Here's how the part is built. I have some questions about the finished solid (model axes, mm). Coordinates: 2 decimals unless noted, no trailing zeros. Write each loop counter-clockwise with the first axis right and the second up, starting at its lowest first coordinate (ties: lowest second). Pieces come first, ordered by that corner, then holes.
Item 1: I want a section at D-D (x = 50). Please give me the cut outline in (y, z), and give its area (3 significant figures).
Item 2: I'm going to push flat-ended pins straight in: P1, Ø3, axis at x = -8.49, y = -8.49, coming from the +Z side; P2, Ø1.5, axis at y = -23, z = 1.5, coming from the +X side; P3, Ø1.5, axis at x = -51, z = 3, coming from the +Y side; P4, Ø2, axis at x = -37.5, z = 3, coming from the -Y side. Where does each tip first touch, or does it pass through?
Item 3: I want a section at A-A (y = 0). Please give me the cut outline in (x, z), and give its area (4 significant figures).
Item 4: I want a section at C-C (y = -50). Please give me the cut outline in (x, z), and give its area (3 significant figures).
Item 5: Please list where these lines run through material, in increasing order: line 1 (Y direction, x = -39.5, z = 4.2); line 2 (Y direction, x = -14, z = 1.35); line 3 (Y direction, x = 1, z = 0.65).
Item 6: I want a section at B-B (x = 0). Please give me the cut outline in (y, z), and give its area (4 significant figures).
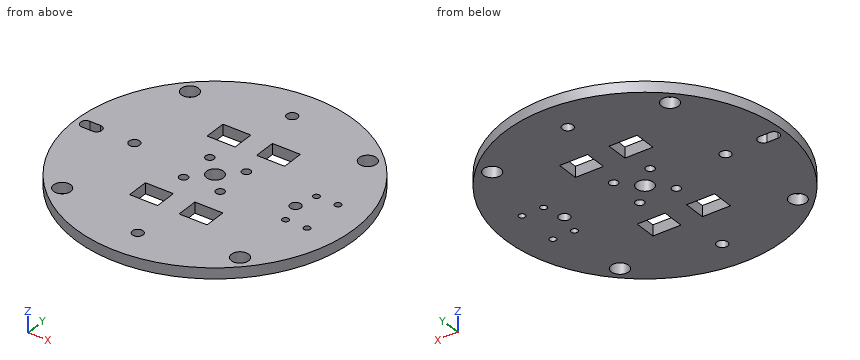
from build123d import *

# Parameters (mm, degrees)
SKETCH1_R           = 65
SKETCH1_R_2         = 2.5
SKETCH1_R_3         = 3.95
SKETCH1_R_4         = 1.5
SKETCH1_R_5         = 4
SKETCH1_R_6         = 2
SKETCH1_W           = 13.02
SKETCH1_H           = 10.2
BOSS_EXTRUDE1_DEPTH = 5


with BuildPart() as part:
    # Sketch1 → Boss-Extrude1 (new body)
    with BuildSketch(Plane.XY):
        Circle(SKETCH1_R)
        with Locations((-37.5, 0)):
            Circle(SKETCH1_R_2, mode=Mode.SUBTRACT)
        with Locations((37.5, 0)):
            Circle(SKETCH1_R_2, mode=Mode.SUBTRACT)
        with Locations((0, 50)):
            Circle(SKETCH1_R_2, mode=Mode.SUBTRACT)
        with Locations((0, -50)):
            Circle(SKETCH1_R_2, mode=Mode.SUBTRACT)
        Circle(SKETCH1_R_3, mode=Mode.SUBTRACT)
        with Locations((50, 10)):
            Circle(SKETCH1_R_4, mode=Mode.SUBTRACT)
        with Locations((50, -10)):
            Circle(SKETCH1_R_4, mode=Mode.SUBTRACT)
        with Locations((40, 10)):
            Circle(SKETCH1_R_4, mode=Mode.SUBTRACT)
        with Locations((40, -10)):
            Circle(SKETCH1_R_4, mode=Mode.SUBTRACT)
        with Locations((-41.365746699, 41.365746699)):
            Circle(SKETCH1_R_5, mode=Mode.SUBTRACT)
        with Locations((41.365746699, -41.365746699)):
            Circle(SKETCH1_R_5, mode=Mode.SUBTRACT)
        with Locations((41.365746699, 41.365746699)):
            Circle(SKETCH1_R_5, mode=Mode.SUBTRACT)
        with Locations((-41.365746699, -41.365746699)):
            Circle(SKETCH1_R_5, mode=Mode.SUBTRACT)
        with Locations((8.485281374, 8.485281374)):
            Circle(SKETCH1_R_6, mode=Mode.SUBTRACT)
        with Locations((8.485281374, -8.485281374)):
            Circle(SKETCH1_R_6, mode=Mode.SUBTRACT)
        with Locations((-8.485281374, -8.485281374)):
            Circle(SKETCH1_R_6, mode=Mode.SUBTRACT)
        with Locations((-8.485281374, 8.485281374)):
            Circle(SKETCH1_R_6, mode=Mode.SUBTRACT)
        with Locations((11.51, -25.1)):
            Rectangle(SKETCH1_W, SKETCH1_H, mode=Mode.SUBTRACT)
        with Locations((-11.51, -25.1)):
            Rectangle(SKETCH1_W, SKETCH1_H, mode=Mode.SUBTRACT)
        with Locations((-11.51, 25.1)):
            Rectangle(SKETCH1_W, SKETCH1_H, mode=Mode.SUBTRACT)
        with Locations((11.51, 25.1)):
            Rectangle(SKETCH1_W, SKETCH1_H, mode=Mode.SUBTRACT)
        with BuildLine():
            Line((-55.056563459, -2.5), (-60.056563459, -2.5))
            ThreePointArc((-60.056563459, -2.5), (-62.556563459, 0), (-60.056563459, 2.5))
            Line((-60.056563459, 2.5), (-55.056563459, 2.5))
            ThreePointArc((-55.056563459, 2.5), (-52.556563459, 0), (-55.056563459, -2.5))
        make_face(mode=Mode.SUBTRACT)
    extrude(amount=BOSS_EXTRUDE1_DEPTH)


solid = part.part
Answer:
1. outline: (-41.53, 0) - (-11.5, 0) - (-11.5, 5) - (-41.53, 5) - close; (-8.5, 0) - (8.5, 0) - (8.5, 5) - (-8.5, 5) - close; (11.5, 0) - (41.53, 0) - (41.53, 5) - (11.5, 5) - close
1. area: 385 mm2
2. P1: passes through
2. P2: stops at x = 61.07
2. P3: stops at y = 41.23
2. P4: stops at y = -53.78
3. outline: (-65, 0) - (-62.56, 0) - (-62.56, 5) - (-65, 5) - close; (-52.56, 0) - (-40, 0) - (-40, 5) - (-52.56, 5) - close; (-35, 0) - (-3.95, 0) - (-3.95, 5) - (-35, 5) - close; (3.95, 0) - (35, 0) - (35, 5) - (3.95, 5) - close; (40, 0) - (65, 0) - (65, 5) - (40, 5) - close
3. area: 510.5 mm2
4. outline: (-41.53, 0) - (-2.5, 0) - (-2.5, 5) - (-41.53, 5) - close; (2.5, 0) - (41.53, 0) - (41.53, 5) - (2.5, 5) - close
4. area: 390 mm2
5. line 1: y = -51.62 to -44.9, -37.83 to -1.5, 1.5 to 37.83, 44.9 to 51.62
5. line 2: y = -63.47 to -30.2, -20 to 20, 30.2 to 63.47
5. line 3: y = -64.99 to -52.29, -47.71 to -3.82, 3.82 to 47.71, 52.29 to 64.99
6. outline: (-65, 0) - (-52.5, 0) - (-52.5, 5) - (-65, 5) - close; (-47.5, 0) - (-3.95, 0) - (-3.95, 5) - (-47.5, 5) - close; (3.95, 0) - (47.5, 0) - (47.5, 5) - (3.95, 5) - close; (52.5, 0) - (65, 0) - (65, 5) - (52.5, 5) - close
6. area: 560.5 mm2
